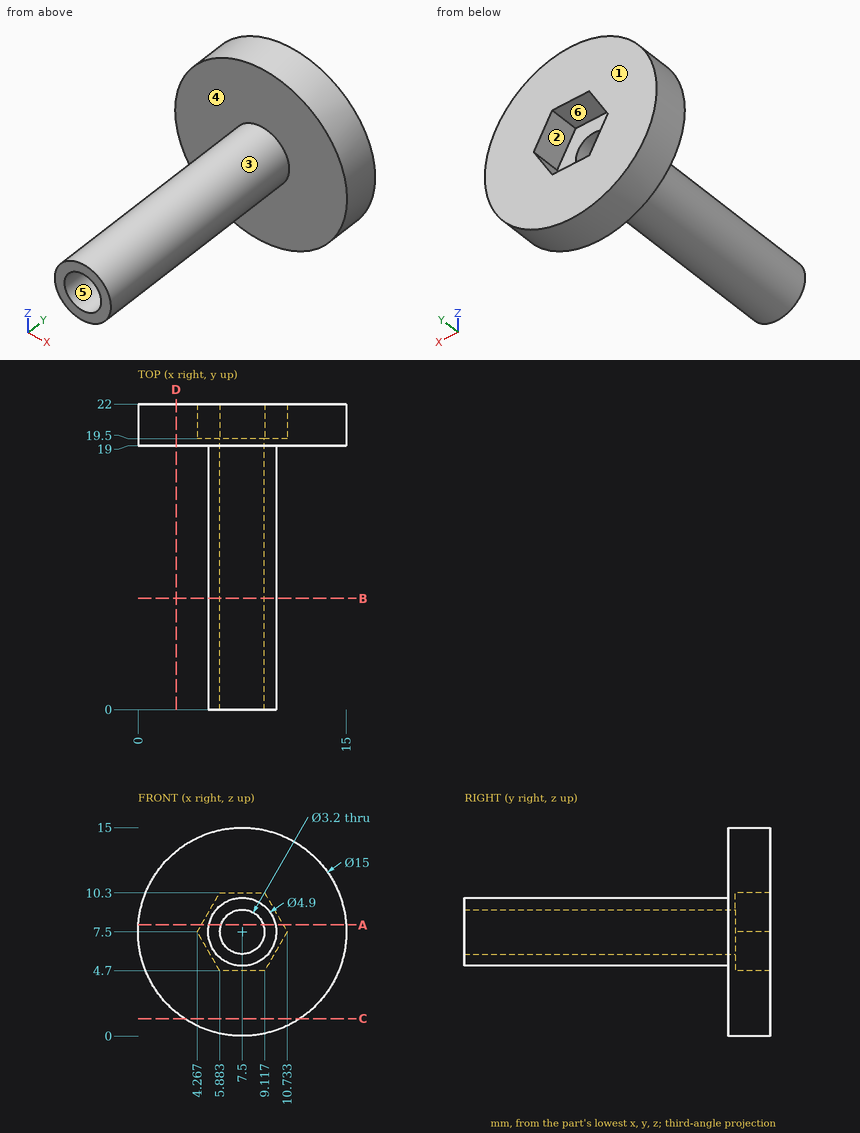
Study the drawing (mm; zero at the part's minimum x, y, z) and answer. A direction names the side the tool comes from. Round coordinates to 2 decimals unless told otherwise and drop trailing zeros. Write each loop counter-clockwise with the first axis right and the second up, starting at its lowest first coordinate (ties: lowest second). Pieces come first, ordered by that corner, then holes.
1) Consider probe 1 along X at (y, z) = (5, 7.5); probe 2 along Y at (x, z) = (5.5, 2); probe 3 along Y at (x, z) = (6, 6). Determine where each line is inside the solid, lowest interval first.
2) Which of the six approach directions +Z, -Z, +X, -X, +Y, -Y give full straight-line access (tool end or side, diameter ignored) to the marked faces 4, 5 and 6?
3) Determine the mould class of the marked faces 1, 2 and 3 for opening direction X: pulls with the +X half, pulls with the -X half, needs draft (parallel to the pull), parting line crosses it, or undercut.
4) Flat-ended cylindrical pins translate along their axes: P1, Ø1.7, axis at x = 8, z = 6.5, coming from the +Y side; P2, Ø6, axis at y = 4.5, z = 11.5, coming from the +X side; P3, Ø1.5, axis at x = 12.5, y = 7, coming from the -Z side; P4, Ø2, axis at x = 4.5, y = 6.5, coming from the -Z side (1 decimal). Find the tip coordinate at first contact, or state that the pin passes through.
5) A cutting plane is placed at A-A on z = 8. Determine the outline of the cut face in (x, y) (1 decimal).
6) A cutting plane is placed at B-B on y = 8. Determine the outline of the cut face in (x, z), and give its area (3 significant figures).
7) A cutting plane is placed at C-C on z = 1.25. Determine the outline of the cut face in (x, y) (1 decimal), and give its area (3 significant figures).
8) A cutting plane is placed at D-D on x = 2.75. Determine the outline of the cut face in (y, z), and give its area (3 significant figures).
Entries:
1. probe 1: x = 5.05 to 5.9, 9.1 to 9.95
1. probe 2: y = 19 to 22
1. probe 3: y = 0 to 19.5
2. face 4: -Y
2. face 5: +Y, -Y
2. face 6: +Y
3. face 1: needs draft
3. face 2: undercut
3. face 3: parting line crosses it
4. P1: stops at y = 19.5
4. P2: stops at x = 9.74
4. P3: passes through
4. P4: stops at z = 6.1
5. outline: (0, 19) - (5.1, 19) - (5.1, 0) - (6, 0) - (6, 19.5) - (4.6, 19.5) - (4.6, 22) - (0, 22) - close; (9, 0) - (9.9, 0) - (9.9, 19) - (15, 19) - (15, 22) - (10.4, 22) - (10.4, 19.5) - (9, 19.5) - close
6. outline: circle Ø4.9 at (7.5, 7.5); hole circle Ø3.2 at (7.5, 7.5)
6. area: 10.8 mm2
7. outline: (3.4, 19) - (11.6, 19) - (11.6, 22) - (3.4, 22) - close
7. area: 24.9 mm2
8. outline: (19, 1.7) - (22, 1.7) - (22, 13.3) - (19, 13.3) - close
8. area: 34.8 mm2
